```python
from build123d import *

# Parameters (mm, degrees)
SKETCH1_R                    = 60
BOSS_EXTRUDE1_DEPTH          = 5
SKETCH2_R                    = 1
CUT_EXTRUDE1_DEPTH           = 5
CHAMFER1_SIZE                = 1
CIRPATTERN1_COUNT            = 4
CHAMFER1_OF_CIRPATTERN1_SIZE = 1
SKETCH3_R                    = 47.75
CUT_EXTRUDE2_DEPTH           = 5


with BuildPart() as part:
    # Sketch1 → Boss-Extrude1 (new body)
    with BuildSketch(Plane(origin=(0, 0, 0), x_dir=(1, 0, 0), z_dir=(0, 1, 0))):
        with Locations(Location((0, 0, 0), (0, 0, 270))):
            Circle(SKETCH1_R)
    extrude(amount=BOSS_EXTRUDE1_DEPTH)

    # Sketch2 → Cut-Extrude1 (cut)
    with BuildSketch(Plane(origin=(0, 5, 0), x_dir=(1, 0, 0), z_dir=(0, 1, 0))):
        with Locations(Location((0, 53.75, 0), (0, 0, 270))):
            Circle(SKETCH2_R)
    cut_extrude1 = extrude(amount=-CUT_EXTRUDE1_DEPTH, mode=Mode.SUBTRACT)

    # Chamfer1
    chamfer1_edges = [part.edges().sort_by_distance(p)[0] for p in [
        (0, 5, -54.75),
    ]]
    chamfer(chamfer1_edges, length=CHAMFER1_SIZE)

    # CirPattern1: Cut-Extrude1 ×4 about axis
    cirpattern1_axis = Axis((0, 0, 0), (0, 1, 0))
    for i in range(1, CIRPATTERN1_COUNT):
        add(cut_extrude1.rotate(cirpattern1_axis, i * 360 / CIRPATTERN1_COUNT), mode=Mode.SUBTRACT)

    # Chamfer1 of CirPattern1
    chamfer1_of_cirpattern1_edges = [part.edges().sort_by_distance(p)[0] for p in [
        (-54.75, 5, 0),
        (0, 5, 54.75),
        (54.75, 5, 0),
    ]]
    chamfer(chamfer1_of_cirpattern1_edges, length=CHAMFER1_OF_CIRPATTERN1_SIZE)

    # Sketch3 → Cut-Extrude2 (cut)
    with BuildSketch(Plane(origin=(0, 5, 0), x_dir=(1, 0, 0), z_dir=(0, 1, 0))):
        with Locations(Location((0, 0, 0), (0, 0, 270))):
            Circle(SKETCH3_R)
    extrude(amount=-CUT_EXTRUDE2_DEPTH, mode=Mode.SUBTRACT)


solid = part.part
```
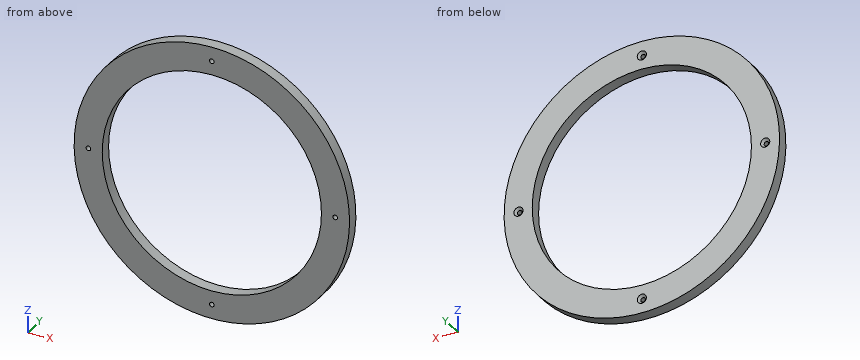
Geometry: final body of the model. Coordinates: model frame, mm. Give positions to 0.01 mm unless a question says otherwise; leave off trailing zeros. Order: outer loops, then holes, each group sorted by start corner. A loop starts at its lowest first (then second) coordinate and runs counter-clockwise, first axis right, second up. Notation, with made-up numbers: (-30.75, 36.5) -> (-11.75, 36.5) arc R35 cw to (-11.75, 72.5) -> close; hole circle Ø7 at (44, 4). An arc over 180 degrees is marked (long way). Write each question's results on one line, items separated by ' | '. Start each with the question number.
1) First-contact query: pin 1 (1.8 mm diameter, centred on x = 0, z = 53.75, fed in from -Y); pin 2 (2.5 mm diameter, centred on x = 0, z = -53.75, fed in from +Y); pin 3 (2 mm diameter, centred on x = -44.5, y = 1.5, fed in from -Z); pin 4 (3 mm diameter, centred on y = 1, z = 11, fed in from +X). Flat tips, straight axial feed; report the tip coordinate or a pass-through.
2) Line query: line 1 (X direction, y = 4.15, z = -41); line 2 (Z direction, x = -8, y = 4.6); line 3 (X direction, y = 1.75, z = -33.5). Output: solid intervals per line, ascending. Write a range as from..to.
3) Section C-C (x = 21). Return loops of the section in (y, z), then the cut area to 3 significant figures.
4) Section B-B (z = -10). Return loops of the section in (x, y).
5) Section A-A (y = 2.3). Return loops of the section in (x, z).
Calculated:
1) pin 1: through | pin 2: y = 4.25 | pin 3: z = -41.32 | pin 4: x = 59.24
2) line 1: -43.81..-24.48, 24.48..43.81 | line 2: -59.46..-47.08, 47.08..59.46 | line 3: -49.78..-34.03, 34.03..49.78
3) outline: (0, -56.2) -> (5, -56.2) -> (5, -42.88) -> (0, -42.88) -> close; (0, 42.88) -> (5, 42.88) -> (5, 56.2) -> (0, 56.2) -> close | area: 133 mm2
4) outline: (-59.16, 0) -> (-46.69, 0) -> (-46.69, 5) -> (-59.16, 5) -> close; (46.69, 0) -> (59.16, 0) -> (59.16, 5) -> (46.69, 5) -> close
5) outline: circle Ø120 at (0, 0); hole circle Ø2 at (-53.75, 0); hole circle Ø95.5 at (0, 0); hole circle Ø2 at (0, -53.75); hole circle Ø2 at (0, 53.75); hole circle Ø2 at (53.75, 0)
